Work out the finished part from the listing and answer in its coordinate system (mm). Face numbers are marked on the shaded views. A direction names the side the tool comes from. Round coordinates to 2 decimals unless told otherwise and drop trailing zeros. Write each loop counter-clockwise with the first axis right and the second up, starting at its lowest first coordinate (ties: lowest second). Pieces come first, ordered by that corner, then holes. Notation, with made-up numbers: M 33,5.5 L 91,5.5 A25 cw 91,25.5 Z; hole C 4,5.25 d7. An arc over 180 degrees is marked long. Answer in a Markdown table with one row per item.
```python
from build123d import *

# Parameters (mm, degrees)
SKETCH1_W           = 55
SKETCH1_H           = 35
SKETCH1_R           = 2
BOSS_EXTRUDE1_DEPTH = 5
SKETCH2_W           = 55
SKETCH2_H           = 30
BOSS_EXTRUDE2_DEPTH = 5
CUT_EXTRUDE1_DEPTH  = 5
FILLET1_R           = 5


with BuildPart() as part:
    # Sketch1 → Boss-Extrude1 (new body)
    with BuildSketch(Plane.XY):
        with Locations((27.5, 17.5)):
            Rectangle(SKETCH1_W, SKETCH1_H)
        with Locations((20, 26.5)):
            Circle(SKETCH1_R, mode=Mode.SUBTRACT)
        with Locations((45, 26.5)):
            Circle(SKETCH1_R, mode=Mode.SUBTRACT)
    extrude(amount=BOSS_EXTRUDE1_DEPTH)

    # Sketch2 → Boss-Extrude2 (add)
    with BuildSketch(Plane.XZ):
        with Locations((27.5, 2.5)):
            Rectangle(SKETCH2_W, SKETCH2_H)
    extrude(amount=BOSS_EXTRUDE2_DEPTH)

    # Sketch5 → Cut-Extrude1 (cut)
    with BuildSketch(Plane.XZ.offset(5)):
        with BuildLine():
            ThreePointArc((17, 12.5), (13.585786438, 13.914213562), (15, 10.5))
            Line((15, 10.5), (15, 12.5))
            Line((15, 12.5), (17, 12.5))
        make_face()
        with BuildLine():
            Line((15, 12.5), (15, 10.5))
            ThreePointArc((15, 10.5), (16.414213562, 11.085786438), (17, 12.5))
            Line((17, 12.5), (15, 12.5))
        make_face()
        with BuildLine():
            ThreePointArc((43, 12.5), (43.585786438, 11.085786438), (45, 10.5))
            Line((45, 10.5), (45, 12.5))
            Line((45, 12.5), (43, 12.5))
        make_face()
        with BuildLine():
            Line((45, 12.5), (45, 10.5))
            ThreePointArc((45, 10.5), (46.414213562, 11.085786438), (47, 12.5))
            ThreePointArc((47, 12.5), (45, 14.5), (43, 12.5))
            Line((43, 12.5), (45, 12.5))
        make_face()
        with BuildLine():
            ThreePointArc((45, -5.5), (43.585786438, -6.085786438), (43, -7.5))
            Line((43, -7.5), (45, -7.5))
            Line((45, -7.5), (45, -5.5))
        make_face()
        with BuildLine():
            Line((45, -7.5), (43, -7.5))
            ThreePointArc((43, -7.5), (45, -9.5), (47, -7.5))
            ThreePointArc((47, -7.5), (46.414213562, -6.085786438), (45, -5.5))
            Line((45, -5.5), (45, -7.5))
        make_face()
        with BuildLine():
            Line((15, -5.5), (15, -7.5))
            Line((15, -7.5), (17, -7.5))
            ThreePointArc((17, -7.5), (16.414213562, -6.085786438), (15, -5.5))
        make_face()
        with BuildLine():
            Line((17, -7.5), (15, -7.5))
            Line((15, -7.5), (15, -5.5))
            ThreePointArc((15, -5.5), (13.585786438, -8.914213562), (17, -7.5))
        make_face()
    extrude(amount=-CUT_EXTRUDE1_DEPTH, mode=Mode.SUBTRACT)

    # Fillet1
    fillet1_edges = [part.edges().sort_by_distance(p)[0] for p in [
        (0, -2.5, 17.5),
        (0, -2.5, -12.5),
        (55, -2.5, -12.5),
        (55, -2.5, 17.5),
        (0, 35, 2.5),
        (55, 35, 2.5),
    ]]
    fillet(fillet1_edges, radius=FILLET1_R)


solid = part.part
```
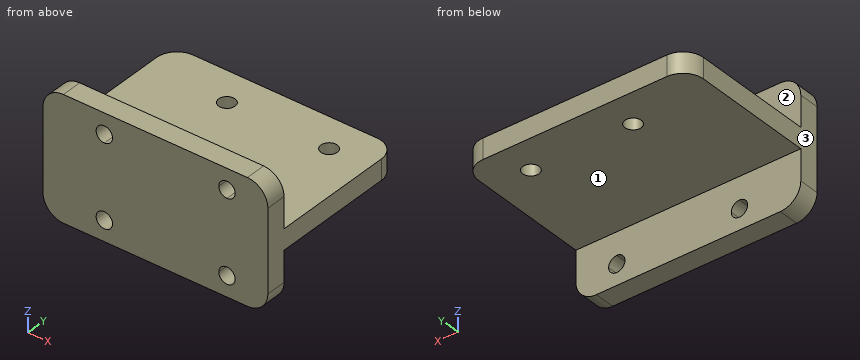
1. The part is cut by section B-B (y = 26.5). Determine the outline of the cut face in (x, z), plus the area to 3 significant figures.
Calculated:
| item | result |
|---|---|
| outline | M 0,0 L 18,0 L 18,5 L 0,5 Z; M 22,0 L 43,0 L 43,5 L 22,5 Z; M 47,0 L 55,0 L 55,5 L 47,5 Z |
| area | 235 mm² |
2. Consider line 1 along Z through (x, y) = (15, -2.7); line 2 along X through (y, z) = (-1.1, 12.5); line 3 along Y through (x, z) = (20, 3.45). Determine where each line is inside the solid, lowest interval first. Write a range as from..to.
Calculated:
| item | result |
|---|---|
| line 1 | z = -12.5..-9.5, -5.5..10.5, 14.5..17.5 |
| line 2 | x = 0..13, 17..43, 47..55 |
| line 3 | y = -5..24.5, 28.5..35 |
3. The part is cut by section A-A (x = 20). Determine the outline of the cut face in (y, z).
Calculated:
| item | result |
|---|---|
| outline | M -5,-12.5 L 0,-12.5 L 0,0 L 24.5,0 L 24.5,5 L 0,5 L 0,17.5 L -5,17.5 Z; M 28.5,0 L 35,0 L 35,5 L 28.5,5 Z |
4. The part is cut by section C-C (z = 4). Determine the outline of the cut face in (x, y), plus the area to 3 significant figures.
Calculated:
| item | result |
|---|---|
| outline | M 0,-5 L 55,-5 L 55,30 A5 ccw 50,35 L 5,35 A5 ccw 0,30 Z; hole C 20,26.5 d4; hole C 45,26.5 d4 |
| area | 2,160 mm² |
5. A tool of negligible diameter and unlimited length cuts with its end or side. For the marked faces 1, 2 and 3, from which of +Z, -Z, +X, -X, +Y, -Y can it reach the whole face along a straight path? Write none if from no direction.
Calculated:
| item | result |
|---|---|
| face 1 | -Z, +X, -X, +Y |
| face 2 | +Z, +X, -X, +Y |
| face 3 | +Z, -Z, -X, +Y, -Y |
6. Given pin 1 (8 mm diameter, centred on y = 28.5, z = -5, fed in from -X); pin 2 (5 mm diameter, centred on x = 15, z = 12.5, fed in from +Y); pin 3 (1.5 mm diameter, centred on x = 30.5, y = 4, fed in from -Z), each flat-ended and moving along its own axis, determine where each tip first touches the part or whether it passes through.
Calculated:
| item | result |
|---|---|
| pin 1 | passes through |
| pin 2 | stops at y = 0 |
| pin 3 | stops at z = 0 |
7. The part is cut by section D-D (x = 42). Determine the outline of the cut face in (y, z), plus the area to 3 significant figures.
Calculated:
| item | result |
|---|---|
| outline | M -5,-12.5 L 0,-12.5 L 0,0 L 35,0 L 35,5 L 0,5 L 0,17.5 L -5,17.5 Z |
| area | 325 mm² |
